Source: CAD feature listing. Evaluate the final solid. Frame: model axes, mm. Face numbers are marked on the shaded views. A direction names the side the tool comes from. Give positions to 0.01 mm unless a question says otherwise; leave off trailing zeros. Order: outer loops, then holes, each group sorted by start corner. A loop starts at its lowest first (then second) coordinate and runs counter-clockwise, first axis right, second up.
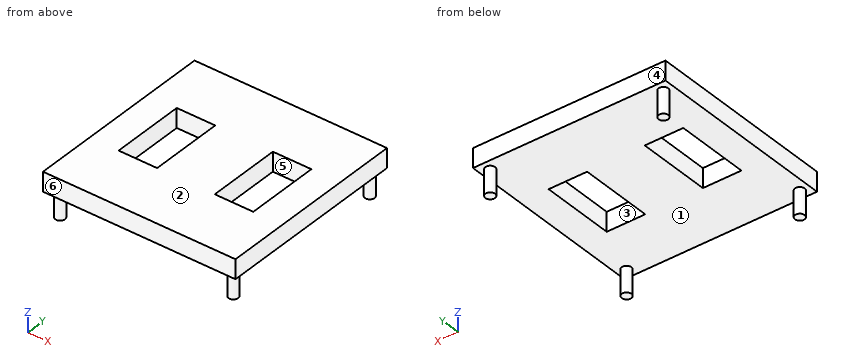
```python
from build123d import *

# Parameters (mm, degrees)
F0_W     = 60
F0_H     = 60
F0_W_2   = 12
F0_H_2   = 23
F1_DEPTH = 6
F2_R     = 1.5
F3_DEPTH = 8


with BuildPart() as f1:
    # F0 (on Top) → F1 (new body)
    with BuildSketch(Plane.XY):
        Rectangle(F0_W, F0_H)
        with Locations((-14.985624, 0)):
            Rectangle(F0_W_2, F0_H_2, mode=Mode.SUBTRACT)
        with Locations((14.985624, 0)):
            Rectangle(F0_W_2, F0_H_2, mode=Mode.SUBTRACT)
    extrude(amount=F1_DEPTH)

    # F2 (on face) → F3 (join)
    with BuildSketch(Plane(origin=(0, 0, 0), x_dir=(1, 0, 0), z_dir=(0, 0, -1))):
        with Locations((-27, 27)):
            Circle(F2_R)
        with Locations((27, 27)):
            Circle(F2_R)
        with Locations((27, -27)):
            Circle(F2_R)
        with Locations((-27, -27)):
            Circle(F2_R)
    extrude(amount=F3_DEPTH)


solid = f1.part
```
1) Reachability of the marked faces 1, 2 and 3 from +Z, -Z, +X, -X, +Y, -Y: full face, straight path, thin tool, end or side. Return the list, or none.
Report:
face 1: -Z
face 2: +Z, +X, -X, +Y, -Y
face 3: +Z, -Z
2) Section query C-C, the plane z = -3.25. Return the cut outline in (x, y).
Report:
outline: circle Ø3 at (-27, -27); circle Ø3 at (-27, 27); circle Ø3 at (27, -27); circle Ø3 at (27, 27)
3) Section query D-D, the plane x = -27. Return the cut outline in (y, z).
Report:
outline: (-30, 0) - (-28.5, 0) - (-28.5, -8) - (-25.5, -8) - (-25.5, 0) - (25.5, 0) - (25.5, -8) - (28.5, -8) - (28.5, 0) - (30, 0) - (30, 6) - (-30, 6) - close
4) Material intervals for L1, parallel to X at y = -3.5, z = 5; L2, parallel to Y at x = 20.5, z = 3.75; L3, parallel to Z at x = -14.5, y = -19, sorted ascending.
Report:
L1: x = -30 to -20.99, -8.99 to 8.99, 20.99 to 30
L2: y = -30 to -11.5, 11.5 to 30
L3: z = 0 to 6
5) Section query A-A, the plane x = 12. Return the cut outline in (y, z), and give its area (3 significant figures).
Report:
outline: (-30, 0) - (-11.5, 0) - (-11.5, 6) - (-30, 6) - close; (11.5, 0) - (30, 0) - (30, 6) - (11.5, 6) - close
area: 222 mm2
6) Draft query along Y for the marked faces 4, 5 and 6. Return one class per face: +Y half, -Y half, draft (parallel to the pull), parting line (faces both ways), or undercut.
Report:
face 4: +Y half
face 5: undercut
face 6: -Y half
7) Section query B-B, the plane y = -10. Return the cut outline in (x, z), and give its area (3 significant figures).
Report:
outline: (-30, 0) - (-20.99, 0) - (-20.99, 6) - (-30, 6) - close; (-8.99, 0) - (8.99, 0) - (8.99, 6) - (-8.99, 6) - close; (20.99, 0) - (30, 0) - (30, 6) - (20.99, 6) - close
area: 216 mm2
8) Pin query (flat end, axial travel): pin 1 (8 mm diameter, centred on y = 4, z = -2, fed in from -X); pin 2 (18 mm diameter, centred on x = 3, y = -8.5, fed in from -Z). Return the tip coordinate at first contact, or that it passes through.
Report:
pin 1: stops at x = -30
pin 2: stops at z = 0
